```python
from build123d import *

# Parameters (mm, degrees)
F0_R            = 82.55
F0_R_2          = 14.1605
F1_DEPTH        = 3.175
F2_R            = 2.3622
F3_DEPTH        = 3.176
F3_COPIES_COUNT = 6


# Not quite as in the source:
# - a pattern or mirror of a feature is missing from the dataset's text; its kind, count and spacing are read off the source's solid


with BuildPart() as f1:
    # F0 (on Top) → F1 (new body)
    with BuildSketch(Plane.XY):
        Circle(F0_R)
        Circle(F0_R_2, mode=Mode.SUBTRACT)
    extrude(amount=F1_DEPTH)

    # F2 (on face) → F3 (cut, through all)
    with BuildSketch(Plane.XY.offset(3.175)):
        with Locations((0, 23.8125)):
            Circle(F2_R)
        with Locations((25.4, 43.9940905122)):
            Circle(F2_R)
    f3 = extrude(amount=-F3_DEPTH, mode=Mode.SUBTRACT)

    # F3_copies: F3 ×6 about axis
    f3_copies_axis = Axis((0, 0, 0), (0, 0, 1))
    for i in range(1, F3_COPIES_COUNT):
        add(f3.rotate(f3_copies_axis, i * 360 / F3_COPIES_COUNT), mode=Mode.SUBTRACT)


solid = f1.part
```
Can you work these out from the model? Positions are in its coordinate system, mm. Coordinates: 2 decimals unless noted, no trailing zeros. Loops run counter-clockwise (first coordinate to the right, second up) from the corner with the lowest first, then second, coordinate; pieces in that order, holes last. Notation, with made-up numbers: M 53.5,-12.5 L 78.5,-12.5 A26 ccw 78.5,25.5 Z; hole C -39,36 d9. An arc over 180 degrees is marked long. Put each result on its own line as item: value. Start each with the question number.
(1) Imagine slicing it at D-D on y = -62. List the corners of the cut face in (x, z) for me (3 decimals).
(2) Will these pins go through, and if not, where does the flat tip stop? pin 1 Ø22.5 at (x, y) = (0, 0) entering from -Z; pin 2 Ø1.5 at (x, z) = (6, 2) entering from +Y.
(3) We'd pull the mould along X, two halves only. Please class faces 1 (the face through (-17.895, -80.587, 1.565)), 2 (the face through (22.875, -11.197, 1.61)), 3 (the face through (-1, -17, 0)): +X half, -X half, draft (parallel to the pull), parting line (faces both ways), or undercut.
(4) I need wall thicknesses on probe 1 along Y at (x, z) = (0, 1.05); probe 2 along X at (y, z) = (-43.5, 0.2); probe 3 along X at (y, z) = (11, 2.1). Which ranges of each line are inside material? Lowest first, please.
(5) Imagine slicing it at A-A on y = 0. Give the number of separate pieces and of enclosed holes in the cut face, and give its area (3 significant figures).
Worked answers:
1. outline: M -54.502,0 L 54.502,0 L 54.502,3.175 L -54.502,3.175 Z
2. pin 1: passes through
2. pin 2: stops at y = 82.38
3. face 1: parting line
3. face 2: undercut
3. face 3: draft
4. probe 1: y = -82.55 to -26.17, -21.45 to -14.16, 14.16 to 21.45, 26.17 to 82.55
4. probe 2: x = -70.16 to -27.71, -23.09 to 23.09, 27.71 to 70.16
4. probe 3: x = -81.81 to -22.8, -18.44 to -8.92, 8.92 to 18.44, 22.8 to 81.81
5. separate pieces: 4
5. enclosed holes: 0
5. area: 404 mm2
